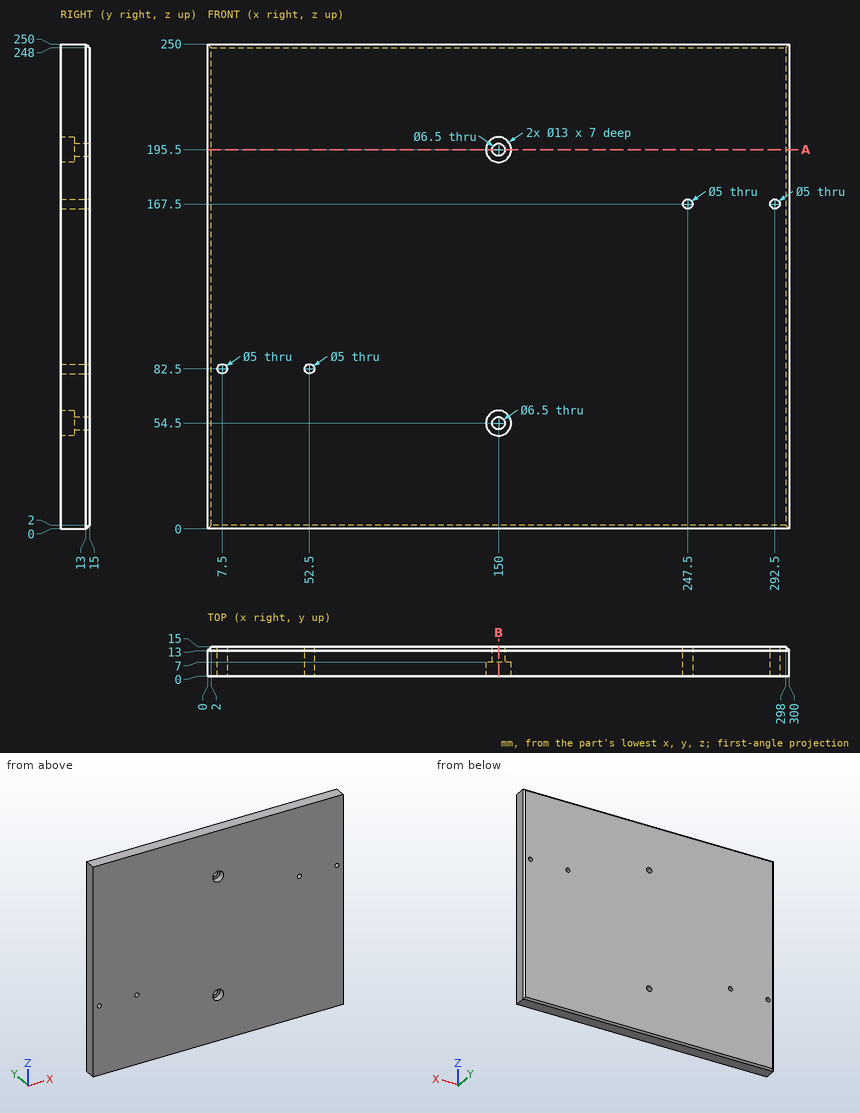
Here's the drawing with two shaded views (mm, measured from the low corner). I have some questions. Coordinates: 2 decimals unless noted, no trailing zeros. Order: outer loops, then holes, each group sorted by start corner. A loop starts at its lowest first (then second) coordinate and runs counter-clockwise, first axis right, second up.
Q1. Will this pin go through, and if not, where does the flat tip stop? pin 1 (6.5 mm diameter, centred on x = 147, z = 195.5, fed in from -Y).
Q2. Suppose I cut it at A-A on z = 195.5. Please give me the cut outline in (x, y), and give its area (3 significant figures).
Q3. Suppose I cut it at B-B on x = 150. Please give me the cut outline in (y, z), and give its area (3 significant figures).
Q4. Please list where these lines run through material, in increasing order: L1, parallel to X at y = 11.5, z = 167.5; L2, parallel to X at y = 4.5, z = 82.5; L3, parallel to Z at x = 150, y = 12.25.
Answer:
1. pin 1: stops at y = 7
2. outline: (0, 0) - (143.5, 0) - (143.5, 7) - (146.75, 7) - (146.75, 15) - (2, 15) - (0, 13) - close; (153.25, 7) - (156.5, 7) - (156.5, 0) - (300, 0) - (300, 13) - (298, 15) - (153.25, 15) - close
2. area: 4,350 mm2
3. outline: (0, 0) - (13, 0) - (15, 2) - (15, 51.25) - (7, 51.25) - (7, 48) - (0, 48) - close; (0, 61) - (7, 61) - (7, 57.75) - (15, 57.75) - (15, 192.25) - (7, 192.25) - (7, 189) - (0, 189) - close; (0, 202) - (7, 202) - (7, 198.75) - (15, 198.75) - (15, 248) - (13, 250) - (0, 250) - close
3. area: 3,460 mm2
4. L1: x = 0 to 245, 250 to 290, 295 to 300
4. L2: x = 0 to 5, 10 to 50, 55 to 300
4. L3: z = 0 to 51.25, 57.75 to 192.25, 198.75 to 250
